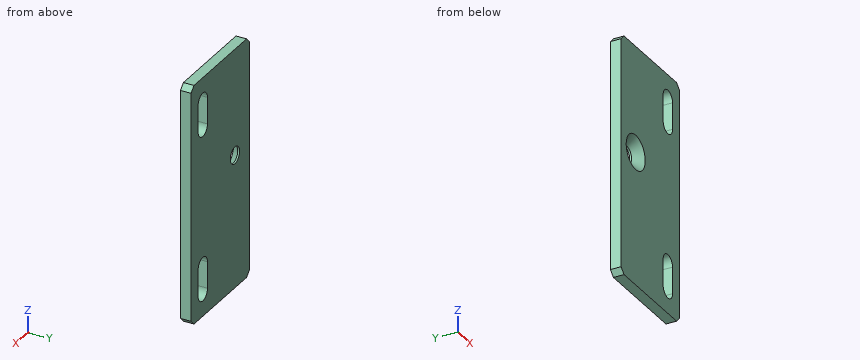
from build123d import *

# Parameters (mm, degrees)
SKETCH1_W        = 20
SKETCH1_H        = 45
BASESHEET_DEPTH  = 2
SCREWSLOTS_DEPTH = 3
CHAMFER1X45_SIZE = 1


with BuildPart() as part:
    # Sketch1 → BaseSheet (new body)
    with BuildSketch(Plane(origin=(0, 0, 0), x_dir=(1, 0, 0), z_dir=(0, 1, 0))):
        Rectangle(SKETCH1_W, SKETCH1_H)
    extrude(amount=BASESHEET_DEPTH)

    # Sketch6 → ScrewSlots (cut, through all)
    with BuildSketch(Plane(origin=(0, 2, 0), x_dir=(1, 0, 0), z_dir=(0, 1, 0))):
        with BuildLine():
            Line((7.6, 18), (7.6, 13))
            ThreePointArc((7.6, 13), (6, 11.4), (4.4, 13))
            Line((4.4, 13), (4.4, 18))
            ThreePointArc((4.4, 18), (6, 19.6), (7.6, 18))
        make_face()
        with BuildLine():
            Line((7.6, -13), (7.6, -18))
            ThreePointArc((7.6, -18), (6, -19.6), (4.4, -18))
            Line((4.4, -18), (4.4, -13))
            ThreePointArc((4.4, -13), (6, -11.4), (7.6, -13))
        make_face()
    extrude(amount=-SCREWSLOTS_DEPTH, mode=Mode.SUBTRACT)

    # Sketch5 → PulleyHole (revolve, cut)
    with BuildSketch(Plane(origin=(-5, 0, 2.5), x_dir=(0, 0, -1), z_dir=(1, 0, 0))):
        Polygon((0, 0), (0, 2), (1.6, 2), (1.6, 1.65), (3.25, 0), align=None)
    revolve(axis=Axis((-5, -6.35, 2.5), (0, 1, 0)), mode=Mode.SUBTRACT)

    # Chamfer1x45
    chamfer1x45_edges = [part.edges().sort_by_distance(p)[0] for p in [
        (-10, 1, -22.5),
        (10, 1, -22.5),
        (10, 1, 22.5),
        (-10, 1, 22.5),
    ]]
    chamfer(chamfer1x45_edges, length=CHAMFER1X45_SIZE)


solid = part.part
The model under review builds one solid part; all positions refer to its coordinate system, in mm. Give positions to 0.01 mm unless a question says otherwise; leave off trailing zeros. Write each loop counter-clockwise with the first axis right and the second up, starting at its lowest first coordinate (ties: lowest second). Pieces come first, ordered by that corner, then holes.
1. Add section B-B, the plane y = 0.85. Write out the cut boundary in (x, z).
2. Wall thickness on L1, parallel to X at y = 1.8, z = 2.5; L2, parallel to Z at x = -5, y = 1.85; L3, parallel to X at y = 1.6, z = -17: over which ranges is each line inside the solid? List them lowest first.
3. Add section A-A, the plane z = 14.5. Write out the cut boundary in (x, y), plus the area to 3 significant figures.
4. Add section D-D, the plane x = -5. Write out the cut boundary in (y, z), plus the area to 3 significant figures.
5. Add section C-C, the plane x = 6. Write out the cut boundary in (y, z), plus the area to 3 significant figures.
6. For P1, Ø5, axis at x = -5, z = 2.5, coming from the -Y side, flat-tipped, find the tip position at first contact; note if it passes through.
Worked answers:
1. outline: (-10, -21.5) - (-9, -22.5) - (9, -22.5) - (10, -21.5) - (10, 21.5) - (9, 22.5) - (-9, 22.5) - (-10, 21.5) - close; hole circle Ø4.8 at (-5, 2.5); hole (4.4, -18) arc R1.6 ccw to (7.6, -18) - (7.6, -13) arc R1.6 ccw to (4.4, -13) - close; hole (4.4, 13) arc R1.6 ccw to (7.6, 13) - (7.6, 18) arc R1.6 ccw to (4.4, 18) - close
2. L1: x = -10 to -6.6, -3.4 to 10
2. L2: z = -22.5 to 0.9, 4.1 to 22.5
2. L3: x = -10 to 4.4, 7.6 to 10
3. outline: (-10, 0) - (4.4, 0) - (4.4, 2) - (-10, 2) - close; (7.6, 0) - (10, 0) - (10, 2) - (7.6, 2) - close
3. area: 33.6 mm2
4. outline: (0, -22.5) - (2, -22.5) - (2, 0.9) - (1.65, 0.9) - (0, -0.75) - close; (0, 5.75) - (1.65, 4.1) - (2, 4.1) - (2, 22.5) - (0, 22.5) - close
4. area: 80.9 mm2
5. outline: (0, -22.5) - (2, -22.5) - (2, -19.6) - (0, -19.6) - close; (0, -11.4) - (2, -11.4) - (2, 11.4) - (0, 11.4) - close; (0, 19.6) - (2, 19.6) - (2, 22.5) - (0, 22.5) - close
5. area: 57.2 mm2
6. P1: stops at y = 0.75
